Part model, mm, in its own coordinate system. Face numbers are marked on the shaded views. Round coordinates to 2 decimals unless told otherwise and drop trailing zeros. Write each loop counter-clockwise with the first axis right and the second up, starting at its lowest first coordinate (ties: lowest second). Pieces come first, ordered by that corner, then holes.
1) Saw through at A-A on x = 8. Write the cut outline in (y, z).
2) Flat gauge pin, fed straight in: pin 1 (2.5 mm diameter, centred on x = 12, z = -6, fed in from +Y). Where does the tip first touch, or does it go through?
3) Saw through at B-B on z = -25. Write the cut outline in (x, y), and give its area (3 significant figures).
4) Pull direction X, two halves, no side cores. Call the marked faces 1, 2 and 3: +X half, -X half, draft (parallel to the pull), parting line (faces both ways), or undercut.
5) Saw through at D-D on y = 1.9. Write the cut outline in (x, z), and give its area (3 significant figures).
6) Drill centre lines: L1, parallel to X at y = 0.35, z = -7; L2, parallel to Z at x = 3.5, y = 0.9; L3, parallel to X at y = 1.2, z = -25. Where is each one in solid material? Low to high.
7) Saw through at C-C on x = 12.75. Write the cut outline in (y, z).
```python
from build123d import *

# Parameters (mm, degrees)
SKETCH1_W           = 16
SKETCH1_H           = 40
SKETCH1_R           = 2.5
BOSS_EXTRUDE1_DEPTH = 3
SKETCH1_3_R         = 1.75
BOSS_EXTRUDE2_DEPTH = 0.5
FILLET1_R           = 0.7


with BuildPart() as part:
    # Sketch1 → Boss-Extrude1 (new body)
    with BuildSketch(Plane(origin=(0, 0, 0), x_dir=(1, 0, 0), z_dir=(0, 1, 0))):
        with Locations((8, 20)):
            Rectangle(SKETCH1_W, SKETCH1_H)
        with Locations(Location((8, 25, 0), (0, 0, 270))):
            Circle(SKETCH1_R, mode=Mode.SUBTRACT)
        with Locations(Location((8, 35, 0), (0, 0, 270))):
            Circle(SKETCH1_R, mode=Mode.SUBTRACT)
        Polygon((14.193375673, 9.5), (11.306624327, 9.5), (9.863248654, 7), (11.306624327, 4.5), (14.193375673, 4.5), (15.636751346, 7), align=None, mode=Mode.SUBTRACT)
        Polygon((6.136751346, 7), (4.693375673, 9.5), (1.806624327, 9.5), (0.363248654, 7), (1.806624327, 4.5), (4.693375673, 4.5), align=None, mode=Mode.SUBTRACT)
    extrude(amount=BOSS_EXTRUDE1_DEPTH)

    # Sketch1_3 → Boss-Extrude2 (add)
    # profile 1 of 2: a face of its own
    with BuildSketch(Plane(origin=(0, 0, 0), x_dir=(1, 0, 0), z_dir=(0, 1, 0))):
        Polygon((4.693375673, 4.5), (6.136751346, 7), (4.693375673, 9.5), (1.806624327, 9.5), (0.363248654, 7), (1.806624327, 4.5), align=None)
        with Locations(Location((3.25, 7, 0), (0, 0, 270))):
            Circle(SKETCH1_3_R, mode=Mode.SUBTRACT)
    # profile 2 of 2: a face of its own
    with BuildSketch(Plane(origin=(0, 0, 0), x_dir=(1, 0, 0), z_dir=(0, 1, 0))):
        Polygon((15.636751346, 7), (14.193375673, 9.5), (11.306624327, 9.5), (9.863248654, 7), (11.306624327, 4.5), (14.193375673, 4.5), align=None)
        with Locations(Location((12.75, 7, 0), (0, 0, 270))):
            Circle(SKETCH1_3_R, mode=Mode.SUBTRACT)
    extrude(amount=BOSS_EXTRUDE2_DEPTH)

    # Fillet1
    fillet1_edges = [part.edges().sort_by_distance(p)[0] for p in [
        (0, 1.5, 0),
        (0, 1.5, -40),
        (16, 1.5, -40),
        (16, 1.5, 0),
    ]]
    fillet(fillet1_edges, radius=FILLET1_R)


solid = part.part
```
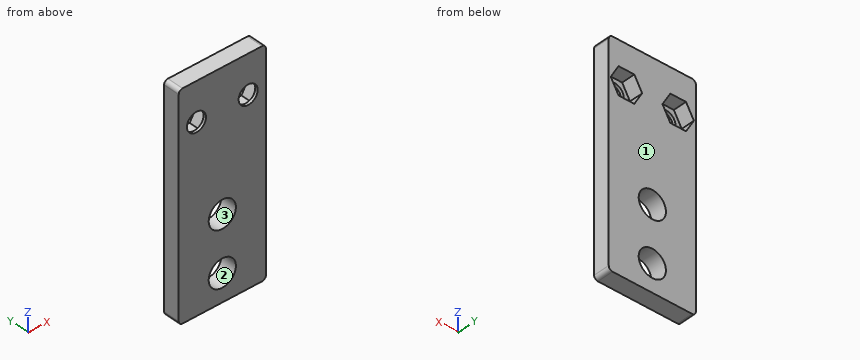
Completed:
1. outline: (0, -40) - (3, -40) - (3, -37.5) - (0, -37.5) - close; (0, -32.5) - (3, -32.5) - (3, -27.5) - (0, -27.5) - close; (0, -22.5) - (3, -22.5) - (3, 0) - (0, 0) - close
2. pin 1: stops at y = 0.5
3. outline: (0, 0) - (5.5, 0) - (5.5, 3) - (0, 3) - close; (10.5, 0) - (16, 0) - (16, 3) - (10.5, 3) - close
3. area: 33.0 mm2
4. face 1: draft
4. face 2: undercut
4. face 3: undercut
5. outline: (0, -39.3) arc R0.7 ccw to (0.7, -40) - (15.3, -40) arc R0.7 ccw to (16, -39.3) - (16, -0.7) arc R0.7 ccw to (15.3, 0) - (0.7, 0) arc R0.7 ccw to (0, -0.7) - close; hole (0.36, -7) - (1.81, -9.5) - (4.69, -9.5) - (6.14, -7) - (4.69, -4.5) - (1.81, -4.5) - close; hole circle Ø5 at (8, -35); hole circle Ø5 at (8, -25); hole (9.86, -7) - (11.31, -9.5) - (14.19, -9.5) - (15.64, -7) - (14.19, -4.5) - (11.31, -4.5) - close
5. area: 557 mm2
6. L1: x = 0 to 1.5, 5 to 11, 14.5 to 16
6. L2: z = -40 to -9.5, -4.5 to 0
6. L3: x = 0 to 5.5, 10.5 to 16
7. outline: (0, -40) - (3, -40) - (3, -9.5) - (0.5, -9.5) - (0.5, -8.75) - (0, -8.75) - close; (0, -5.25) - (0.5, -5.25) - (0.5, -4.5) - (3, -4.5) - (3, 0) - (0, 0) - close
